from build123d import *

# Parameters (mm, degrees)
F0_R     = 3.25
F1_DEPTH = 4.15


with BuildPart() as f1:
    # F0 (on Right) → F1 (new body)
    with BuildSketch(Plane.YZ):
        with BuildLine():
            Line((-13.613708, 0), (0, 0))
            Line((0, 0), (0, 4))
            Line((0, 4), (8, 4))
            Line((8, 4), (8, 12))
            Line((8, 12), (0, 12))
            Line((0, 12), (0, 16))
            Line((0, 16), (8, 16))
            Line((8, 16), (8, 24))
            Line((8, 24), (0, 24))
            Line((0, 24), (0, 28))
            Line((0, 28), (8, 28))
            Line((8, 28), (8, 36))
            Line((8, 36), (0, 36))
            Line((0, 36), (0, 40))
            Line((0, 40), (-19.919684, 40))
            ThreePointArc((-19.919684, 40), (-21.832713, 38.597309), (-21.070201, 36.351023))
            Line((-21.070201, 36.351023), (-12, 30))
            Line((-12, 30), (-21.070201, 23.648977))
            ThreePointArc((-21.070201, 23.648977), (-26.012028, 9.090825), (-13.613708, 0))
        make_face()
        with Locations((-10.754399, 13.5)):
            Circle(F0_R, mode=Mode.SUBTRACT)
        with Locations((-6.143649, 33.287299)):
            Circle(F0_R, mode=Mode.SUBTRACT)
    extrude(amount=F1_DEPTH)


solid = f1.part
Input: part model. Units: mm. Frame: model coordinates. A direction names the side the tool comes from. Round coordinates to 2 decimals unless told otherwise and drop trailing zeros. Loops run counter-clockwise (first coordinate to the right, second up) from the corner with the lowest first, then second, coordinate; pieces in that order, holes last. Notation, with made-up numbers: (45.25, 5) -> (75.25, 5) arc R26 cw to (75.25, 21) -> close; hole circle Ø6 at (77.5, -28.75). An arc over 180 degrees is marked (long way). Answer as a JSON object with one key per item and string values. Group by question number.
1) Draft query along Y for faces 1 (the cylindrical face through (2.05, -21.82, 38.63)), 2 (the flat face through (2, -10, 40)), 3 (the cylindrical face through (2.046, -6.848, 30.115)). Return one class per face: +Y half, -Y half, draft (parallel to the pull), parting line (faces both ways), or undercut.
2) Reachability of faces 4 (the flat face through (2, 8, 8)), 5 (the flat face through (0, -10, 20)), 6 (the flat face through (2, 0, 26)), 7 (the flat face through (2.05, -16.6, 33.22)), 8 (the flat face through (2, 4, 36)) from +Z, -Z, +X, -X, +Y, -Y: full face, straight path, thin tool, end or side. Return the list, or none.
3) Ray query, L1, parallel to Z at x = 0.95, y = 6.5; L2, parallel to Y at x = 3.45, z = 11.5; L3, parallel to Y at x = 1.1, z = 35. Return the intervals inside material, ascending.
4) Pin query (flat end, axial travel): pin 1 (2 mm diameter, centred on x = 3, z = 1.5, fed in from +Y); pin 2 (2 mm diameter, centred on x = 3, y = 4, fed in from +Z); pin 3 (6 mm diameter, centred on y = -10.75, z = 13.5, fed in from -X); pin 4 (2 mm diameter, centred on x = 1, z = 31, fed in from -Y). Return the tip coordinate at first contact, or that it passes through.
5) Section query B-B on z = 13.5. Output: boundary loops of the cut face in (x, y).
6) Section query A-A on y = -18. Output: boundary loops of the cut face in (x, z).
7) Section query C-C on x = 0.7. Output: boundary loops of the cut face in (y, z), plus the area to 3 significant figures.
8) Section query D-D on z = 22. Output: boundary loops of the cut face in (x, y).
Reply:
{
 "1": {"face 1": "-Y half", "face 2": "draft", "face 3": "undercut"},
 "2": {"face 4": "+Z, -Z, +X, -X, +Y", "face 5": "+Z, -Z, -X, +Y, -Y", "face 6": "+X, -X, +Y", "face 7": "+X, -X, -Y", "face 8": "+Z, +X, -X, +Y"},
 "3": {"L1": "z = 4 to 12, 16 to 24, 28 to 36", "L2": "y = -26.53 to -13.32, -8.19 to 8", "L3": "y = -19.14 to -8.91, -3.38 to 8"},
 "4": {"pin 1": "stops at y = 0", "pin 2": "stops at z = 36", "pin 3": "passes through", "pin 4": "stops at y = -14.86"},
 "5": {"outline": "(0, -26.6) -> (4.15, -26.6) -> (4.15, -14) -> (0, -14) -> close; (0, -7.5) -> (4.15, -7.5) -> (4.15, 0) -> (0, 0) -> close"},
 "6": {"outline": "(0, 0.76) -> (4.15, 0.76) -> (4.15, 25.8) -> (0, 25.8) -> close; (0, 34.2) -> (4.15, 34.2) -> (4.15, 40) -> (0, 40) -> close"},
 "7": {"outline": "(-21.07, 23.65) arc R13 ccw to (-13.61, 0) -> (0, 0) -> (0, 4) -> (8, 4) -> (8, 12) -> (0, 12) -> (0, 16) -> (8, 16) -> (8, 24) -> (0, 24) -> (0, 28) -> (8, 28) -> (8, 36) -> (0, 36) -> (0, 40) -> (-19.92, 40) arc R2.01 ccw to (-21.07, 36.35) -> (-12, 30) -> close; hole circle Ø6.5 at (-10.75, 13.5); hole circle Ø6.5 at (-6.14, 33.29)", "area": "990 mm2"},
 "8": {"outline": "(0, -22.99) -> (4.15, -22.99) -> (4.15, 8) -> (0, 8) -> close"}
}
